Build history of the part. All positions in model axes, mm. A direction names the side the tool comes from. Round coordinates to 2 decimals unless told otherwise and drop trailing zeros. Write each loop counter-clockwise with the first axis right and the second up, starting at its lowest first coordinate (ties: lowest second). Pieces come first, ordered by that corner, then holes. Notation, with made-up numbers: (39.25, -18) - (86.25, -18) arc R25 cw to (86.25, 7) - close; hole circle Ø7 at (14, -23.75). An arc over 180 degrees is marked (long way). One line per question, with ' | ' between items.
from build123d import *

# Parameters (mm, degrees)
BOSS_EXTRUDE1_DEPTH = 100
SKETCH2_W           = 50
SKETCH2_H           = 30
BOSS_EXTRUDE2_DEPTH = 30
SKETCH4_W           = 50
SKETCH4_H           = 40
CUT_EXTRUDE2_DEPTH  = 188.082869339


with BuildPart() as part:
    # Sketch1 → Boss-Extrude1 (new body)
    with BuildSketch(Plane.XY):
        Polygon((0, 0), (0, 50), (50, 50), (50, 80), (80, 80), (150, 40), (150, 0), align=None)
    extrude(amount=BOSS_EXTRUDE1_DEPTH)

    # Sketch2 → Boss-Extrude2 (add)
    with BuildSketch(Plane(origin=(0, 80, 0), x_dir=(1, 0, 0), z_dir=(0, 1, 0))):
        with Locations((25, -55)):
            Rectangle(SKETCH2_W, SKETCH2_H)
    extrude(amount=-BOSS_EXTRUDE2_DEPTH)

    # Sketch4 → Cut-Extrude2 (cut, through all)
    with BuildSketch(Plane(origin=(0, 50, 0), x_dir=(1, 0, 0), z_dir=(0, 1, 0))):
        with Locations((25, -20)):
            Rectangle(SKETCH4_W, SKETCH4_H)
    extrude(amount=-CUT_EXTRUDE2_DEPTH, mode=Mode.SUBTRACT)


solid = part.part
Q1. Drop flat-ended pins along their axis: pin 1 (10 mm diameter, centred on x = 135, z = 37.5, fed in from +Y); pin 2 (5 mm diameter, centred on y = 63.5, z = 11.5, fed in from +X); pin 3 (8 mm diameter, centred on x = 85.5, z = 22, fed in from -Y); pin 4 (6 mm diameter, centred on y = 45, z = 25, fed in from -X). Give the stop position or say it passes through.
Found:
pin 1: y = 51.43 | pin 2: x = 113.25 | pin 3: y = 0 | pin 4: x = 50
Q2. Which spindle directions (+Z, -Z, +X, -X, +Y, -Y) get a long thin tool onto all of the face, cutting with end or side? Do faces 1 (the flat face through (76, 32, 100)), 2 (the flat face through (50, 65, 85)), 3 (the flat face through (25, 41, 40)). Say none if no direction does.
Found:
face 1: +Z, +X, -X, +Y, -Y | face 2: +Z, -X, +Y | face 3: -Z, -X, +Y, -Y
Q3. Saw through at A-A, the plane y = 52. List the corners of the cut face in (x, z).
Found:
outline: (0, 40) - (50, 40) - (50, 0) - (129, 0) - (129, 100) - (50, 100) - (50, 70) - (0, 70) - close
Q4. Saw through at C-C, the plane x = 22.5. List the corners of the cut face in (y, z), then the cut area to 3 significant figures.
Found:
outline: (0, 40) - (80, 40) - (80, 70) - (50, 70) - (50, 100) - (0, 100) - close | area: 3,900 mm^2
Q5. Saw through at B-B, the plane z = 57. List the corners of the cut face in (x, y).
Found:
outline: (0, 0) - (150, 0) - (150, 40) - (80, 80) - (0, 80) - close
Q6. Drill centre lines: L1, parallel to Y at x = 46, z = 85.5; L2, parallel to X at y = 33.5, z = 33.5; L3, parallel to Y at x = 129.5, z = 39.5. Where is each one in solid material? Low to high. Write a range as from..to.
Found:
L1: 0..50 | L2: 50..150 | L3: 0..51.71
Q7. Saw through at D-D, the plane z = 35. List the corners of the cut face in (x, y), then the cut area to 3 significant figures.
Found:
outline: (50, 0) - (150, 0) - (150, 40) - (80, 80) - (50, 80) - close | area: 6,600 mm^2
